The listing builds one solid part. Answer for the finished solid, in the listing's coordinates (mm). A direction names the side the tool comes from. Give positions to 0.01 mm unless a question says otherwise; leave off trailing zeros. Loops run counter-clockwise (first coordinate to the right, second up) from the corner with the lowest first, then second, coordinate; pieces in that order, holes last. Notation, with made-up numbers: M 29,4 L 59,4 A14 cw 59,15 Z; hole C 35.25,60 d5. An arc over 180 degrees is marked long. Return JSON: item names as keys, results as strings.
from build123d import *

# Parameters (mm, degrees)
SKETCH1_W           = 18.250795329
SKETCH1_H           = 3
BOSS_EXTRUDE1_DEPTH = 15


with BuildPart() as part:
    # Sketch1 → Boss-Extrude1 (new, symmetric)
    with BuildSketch(Plane.XY):
        Polygon((3, 0), (0, 0), (0, 42), (12.496402878, 42), (12.496402878, 39), (3, 39), align=None)
        with Locations((12.125397665, 1.5)):
            Rectangle(SKETCH1_W, SKETCH1_H)
    extrude(amount=BOSS_EXTRUDE1_DEPTH, both=True)


solid = part.part
(1) The part is cut by section A-A (x = 6.5). Determine the outline of the cut face in (y, z), and give its area (3 significant figures).
Values follow:
{"outline": "M 0,-15 L 3,-15 L 3,15 L 0,15 Z; M 39,-15 L 42,-15 L 42,15 L 39,15 Z", "area": "180 mm²"}
(2) Given pin 1 (0.9 mm diameter, centred on y = 41, z = -0.5, fed in from +X); pin 2 (6 mm diameter, centred on x = 4.5, z = -4.5, fed in from -Y); pin 3 (4 mm diameter, centred on y = 8.5, z = 7, fed in from +X), each flat-ended and moving along its own axis, determine where each tip first touches the part or whether it passes through.
Values follow:
{"pin 1": "x = 12.5", "pin 2": "y = 0", "pin 3": "x = 3"}
(3) Determine the mould class of faces 4 (the flat face through (10, 0, 0)), 5 (the flat face through (12, 3, 0)), 6 (the flat face through (2.8, 18, -15)) for opening direction Y: released by +Y, released by -Y, zero draft, split by the parting line, or undercut.
Values follow:
{"face 4": "released by -Y", "face 5": "undercut", "face 6": "zero draft"}
(4) Straight lines are drawn through the part: line 1 along Y through (x, z) = (10.25, -8.5); line 2 along X through (y, z) = (30.5, 0). For each, find the intervals that lie inside material, in ascending order.
Values follow:
{"line 1": "0 to 3, 39 to 42", "line 2": "0 to 3"}
(5) A tool of negligible diameter and unlimited length cuts with its end or side. For faces 1 (the flat face through (8, 39, 0)), 2 (the flat face through (6, 42, 0)), 3 (the flat face through (12.496, 41, 0)), from which of +Z, -Z, +X, -X, +Y, -Y can it reach the whole face along a straight path? Write none if from no direction.
Values follow:
{"face 1": "+Z, -Z, +X", "face 2": "+Z, -Z, +X, -X, +Y", "face 3": "+Z, -Z, +X, +Y"}
(6) The part is cut by section C-C (y = 24). Determine the outline of the cut face in (x, z), and give its area (3 significant figures).
Values follow:
{"outline": "M 0,-15 L 3,-15 L 3,15 L 0,15 Z", "area": "90.0 mm²"}
(7) The part is cut by section B-B (z = 9.25). Determine the outline of the cut face in (x, y).
Values follow:
{"outline": "M 0,0 L 21.25,0 L 21.25,3 L 3,3 L 3,39 L 12.5,39 L 12.5,42 L 0,42 Z"}
